```python
from build123d import *

# Parameters (mm, degrees)
SKETCH1_R           = 3
BOSS_EXTRUDE2_DEPTH = 30
SHELL1_T            = -3
SKETCH3_R           = 1.75
BOSS_EXTRUDE3_DEPTH = 10
SKETCH5_R           = 1.65
BOSS_EXTRUDE4_DEPTH = 3
CUT_EXTRUDE1_START  = -27
CUT_EXTRUDE1_DEPTH  = 27
CUT_EXTRUDE2_START  = -3
CUT_EXTRUDE2_DEPTH  = 3
BOSS_EXTRUDE5_START = -3
SKETCH8_R           = 1.65
BOSS_EXTRUDE5_DEPTH = 3
SKETCH9_R           = 1
CUT_EXTRUDE3_DEPTH  = 30


with BuildPart() as part:
    # Sketch1 → Boss-Extrude2 (new body)
    with BuildSketch(Plane.XY):
        with BuildLine():
            Line((-12.3, -61.113910037), (-12.3, 61.113910037))
            ThreePointArc((-12.3, 61.113910037), (-17.145844754, 58.748987809), (-16.028571429, 64.024096229))
            Line((-16.028571429, 64.024096229), (-16.757142857, 66.934282421))
            ThreePointArc((-16.757142857, 66.934282421), (-69, 0), (-16.757142857, -66.934282421))
            Line((-16.757142857, -66.934282421), (-16.028571429, -64.024096229))
            ThreePointArc((-16.028571429, -64.024096229), (-17.145844754, -58.748987809), (-12.3, -61.113910037))
        make_face()
        with Locations((-63, 0)):
            Circle(SKETCH1_R, mode=Mode.SUBTRACT)
    extrude(amount=BOSS_EXTRUDE2_DEPTH)

    # Shell1
    shell1_openings = [part.faces().sort_by_distance(p)[0] for p in [
        (-36.229379507, 0, 30),
    ]]
    offset(amount=SHELL1_T, openings=shell1_openings)

    # Sketch3 → Boss-Extrude3 (add)
    with BuildSketch(Plane.YZ.offset(-12.3)):
        with Locations(Location((15, 4, 0), (0, 0, 180))):
            Circle(SKETCH3_R)
    extrude(amount=BOSS_EXTRUDE3_DEPTH)

    # Sketch5 → Boss-Extrude4 (add)
    with BuildSketch(Plane.XY):
        with BuildLine():
            Line((-12.3, -61.113910037), (-12.3, 61.113910037))
            ThreePointArc((-12.3, 61.113910037), (-13.454155246, 63.478832265), (-16.028571429, 64.024096229))
            Line((-16.028571429, 64.024096229), (-16.757142857, 66.934282421))
            ThreePointArc((-16.757142857, 66.934282421), (-69, 0), (-16.757142857, -66.934282421))
            Line((-16.757142857, -66.934282421), (-16.028571429, -64.024096229))
            ThreePointArc((-16.028571429, -64.024096229), (-13.454155246, -63.478832265), (-12.3, -61.113910037))
        make_face()
        with Locations((-63, 0)):
            Circle(SKETCH5_R, mode=Mode.SUBTRACT)
        with Locations((-15.3, 61.113910037)):
            Circle(SKETCH5_R, mode=Mode.SUBTRACT)
        with Locations((-15.3, -61.113910037)):
            Circle(SKETCH5_R, mode=Mode.SUBTRACT)
    extrude(amount=BOSS_EXTRUDE4_DEPTH)

    # Sketch6 → Cut-Extrude1 (cut)
    with BuildSketch(Plane.XY.offset(30).offset(CUT_EXTRUDE1_START)):
        with BuildLine():
            Line((-63, 3), (-68.934751758, 3))
            ThreePointArc((-68.934751758, 3), (-71.934751758, 0), (-68.934751758, -3))
            Line((-68.934751758, -3), (-63, -3))
            ThreePointArc((-63, -3), (-60, 0), (-63, 3))
        make_face()
        with BuildLine():
            Line((-14.571428571, -58.203723845), (-12.3, -58.772380917))
            Line((-12.3, -58.772380917), (-12.3, -61.113910037))
            ThreePointArc((-12.3, -61.113910037), (-12.935077772, -59.268065283), (-14.571428571, -58.203723845))
        make_face()
        with BuildLine():
            Line((-14.571428571, 58.203723845), (-12.3, 58.772380917))
            Line((-12.3, 58.772380917), (-12.3, 61.113910037))
            ThreePointArc((-12.3, 61.113910037), (-12.935077772, 59.268065283), (-14.571428571, 58.203723845))
        make_face()
    extrude(amount=CUT_EXTRUDE1_DEPTH, mode=Mode.SUBTRACT)

    # Sketch7 → Cut-Extrude2 (cut)
    with BuildSketch(Plane.XY.offset(30).offset(CUT_EXTRUDE2_START)):
        Polygon((-13.596816706, -58.163910037), (-11.893633412, -58.163910037), (-11.893633412, -61.113910037), (-13.596816706, -64.063910037), (-17.003183294, -64.063910037), (-18.706366588, -61.113910037), (-17.003183294, -58.163910037), align=None)
        Polygon((-11.893633412, 61.113910037), (-13.596816706, 64.063910037), (-17.003183294, 64.063910037), (-18.706366588, 61.113910037), (-17.003183294, 58.163910037), (-13.596816706, 58.163910037), (-11.893633412, 58.163910037), align=None)
        Polygon((-59.593633412, 0), (-61.296816706, 2.95), (-64.703183294, 2.95), (-66.406366588, 0), (-64.703183294, -2.95), (-61.296816706, -2.95), align=None)
    extrude(amount=-CUT_EXTRUDE2_DEPTH, mode=Mode.SUBTRACT)

    # Sketch8 → Boss-Extrude5 (add)
    # profile 1 of 3: a face of its own
    with BuildSketch(Plane.XY.offset(30).offset(BOSS_EXTRUDE5_START)):
        with BuildLine():
            Line((-63, 3), (-68.934751758, 3))
            Line((-68.934751758, 3), (-68.934751758, -3))
            Line((-68.934751758, -3), (-63, -3))
            ThreePointArc((-63, -3), (-60, 0), (-63, 3))
        make_face()
        with Locations((-63, 0)):
            Circle(SKETCH8_R, mode=Mode.SUBTRACT)
    # profile 2 of 3: a face of its own
    with BuildSketch(Plane.XY.offset(30).offset(BOSS_EXTRUDE5_START)):
        with BuildLine():
            Line((-12.3, -58.772380917), (-14.571428571, -58.203723845))
            ThreePointArc((-14.571428571, -58.203723845), (-17.664922228, -62.959754791), (-12.3, -61.113910037))
            Line((-12.3, -61.113910037), (-12.3, -58.772380917))
        make_face()
        with Locations((-15.3, -61.113910037)):
            Circle(SKETCH8_R, mode=Mode.SUBTRACT)
    # profile 3 of 3: a face of its own
    with BuildSketch(Plane.XY.offset(30).offset(BOSS_EXTRUDE5_START)):
        with BuildLine():
            Line((-12.3, 61.113910037), (-12.3, 58.772380917))
            Line((-12.3, 58.772380917), (-14.571428571, 58.203723845))
            ThreePointArc((-14.571428571, 58.203723845), (-17.664922228, 62.959754791), (-12.3, 61.113910037))
        make_face()
        with Locations((-15.3, 61.113910037)):
            Circle(SKETCH8_R, mode=Mode.SUBTRACT)
    extrude(amount=BOSS_EXTRUDE5_DEPTH)

    # Sketch9 → Cut-Extrude3 (cut)
    with BuildSketch(Plane.YZ.offset(-2.3)):
        with Locations((15, 4)):
            Circle(SKETCH9_R)
    extrude(amount=-CUT_EXTRUDE3_DEPTH, mode=Mode.SUBTRACT)


solid = part.part
```
Here's how the part is built. I have some questions about the finished solid (model axes, mm). A direction names the side the tool comes from. Give positions to 0.01 mm unless a question says otherwise; leave off trailing zeros. Write each loop counter-clockwise with the first axis right and the second up, starting at its lowest first coordinate (ties: lowest second). Pieces come first, ordered by that corner, then holes. Notation, with made-up numbers: (75.25, 38.5) -> (131.25, 38.5) arc R11 cw to (131.25, 58.5) -> close; hole circle Ø2 at (-39, 58). An arc over 180 degrees is marked (long way). Use one line per item in the form item = value.
1) Suppose I cut it at C-C (x = -9.5). Please give me the cut outline in (y, z).
Verdict:
outline = circle Ø3.5 at (15, 4); hole circle Ø2 at (15, 4)
2) Suppose I cut it at B-B (x = -43.5). Please give me the cut outline in (y, z), and give its area (3 significant figures).
Verdict:
outline = (-53.56, 0) -> (53.56, 0) -> (53.56, 30) -> (49.64, 30) -> (49.64, 3) -> (-49.64, 3) -> (-49.64, 30) -> (-53.56, 30) -> close
area = 533 mm2
3) I'm going to push flat-ended pins straight in: pin 1 (2.5 mm diameter, centred on x = -15.3, y = 61.11, fed in from -Z); pin 2 (1 mm diameter, centred on x = -34.5, y = -42.5, fed in from +Z); pin 3 (12 mm diameter, centred on y = -6, z = 9, fed in from -X); pin 4 (1 mm diameter, centred on y = -23.5, z = 15, fed in from -X). Where does each tip first touch, or does it pass through?
Verdict:
pin_1 = through
pin_2 = 3
pin_3 = -68.93
pin_4 = -65.05
4) Suppose I cut it at D-D (y = -29). Please give me the cut outline in (x, z), and give its area (3 significant figures).
Verdict:
outline = (-62.61, 0) -> (-12.3, 0) -> (-12.3, 30) -> (-15.3, 30) -> (-15.3, 3) -> (-59.29, 3) -> (-59.29, 30) -> (-62.61, 30) -> close
area = 322 mm2
5) If I drill on L1, parallel to Y at x = -15.3, z = 2.2; L2, parallel to Y at x = -6.5, z = 4; L3, parallel to Z at x = -45.5, y = -22.5, over which ranges is the centre line in solid material (lowest first)? Write a range as [from, to].
Verdict:
L1 = [-64.11, -62.76], [-59.46, 59.46], [62.76, 64.11]
L2 = [13.25, 14], [16, 16.75]
L3 = [0, 3]
6) Suppose I cut it at A-A (z = 20.75). Please give me the cut outline in (x, y), and give its area (3 significant figures).
Verdict:
outline = (-68.93, -3) arc R69 ccw to (-16.76, -66.93) -> (-16.03, -64.02) arc R3 cw to (-14.57, -58.2) -> (-12.3, -58.77) -> (-12.3, 58.77) -> (-14.57, 58.2) arc R3 cw to (-16.03, 64.02) -> (-16.76, 66.93) arc R69 ccw to (-68.93, 3) -> (-63, 3) arc R3 cw to (-63, -3) -> close; hole (-65.79, -5.31) arc R66 ccw to (-21.13, -62.53) arc R6 cw to (-15.3, -55.11) -> (-15.3, 55.11) arc R6 cw to (-21.13, 62.53) arc R66 ccw to (-65.79, 5.31) arc R6 cw (long way) to start
area = 983 mm2
7) We'd pull the mould along Y, two halves only. Please class faces 1 (the face through (-13.48, -63.5, 1.48)), 2 (the face through (-2.3, 14, 5)), 3 (the face through (-20.06, -57.46, 16.31)): +Y half, -Y half, draft (parallel to the pull), parting line (faces both ways), or undercut.
Verdict:
face_1 = -Y half
face_2 = draft
face_3 = undercut
8) On a 3-axis mill with a long thin cutter (end or side, diameter ignored), from which of +Z, -Z, +X, -X, +Y, -Y can I reach the whole of each face in a straight line? I mean faces 4 (the face through (-15.515, -59.478, 1.479)), 5 (the face through (-35, 1, 0)), 6 (the face through (-14, -58.164, 26)), 7 (the face through (-15.3, -1, 16)), 8 (the face through (-65, 0, 27)). Say none if no direction works.
Verdict:
face_4 = +Z, -Z
face_5 = -Z, +X, -X, +Y, -Y
face_6 = +X, -Y
face_7 = +Z
face_8 = -X
